Verification items for the finished model (mm, model axes). A direction names the side the tool comes from. Give positions to 0.01 mm unless a question says otherwise; leave off trailing zeros. Order: outer loops, then holes, each group sorted by start corner. A loop starts at its lowest first (then second) coordinate and runs counter-clockwise, first axis right, second up. Notation, with made-up numbers: (29, -31.75) -> (46, -31.75) arc R24 cw to (46, 6.25) -> close; hole circle Ø1 at (81, 78). An arc over 180 degrees is marked (long way). Return JSON: item names as keys, results as strings. Group by question number.
(1) Cross-section at C-C on x = 26.75. Enter the section's corners in (y, z).
(2) Cross-section at D-D on y = 14.5. Enter the section's corners in (x, z).
(3) Cross-section at A-A on x = 14.3. Enter the section's corners in (y, z).
(4) Depth check by flat-ended pin: pin 1 Ø9.5 at (x, z) = (17, 26) entering from -Y; pin 2 Ø3.5 at (x, y) = (11, 15) entering from +Z; pin 3 Ø6 at (x, z) = (10.5, 26) entering from +Y. Enter the tip coordinate at first touch or a pass-through.
(5) Tool access check on faces 1 (the face through (11.1, 10.4, -4.9)), 2 (the face through (14, 13, 26)), 3 (the face through (14, 8, -10)), 4 (the face through (14, 2, 20)). Record the directions out of +Z, -Z, +X, -X, +Y, -Y that give a thin tool (end or side, any length) a straight path to the whole face; none if there is none.
(6) Cross-section at B-B on y = 8. Enter the section's corners in (x, z), then the cut area to 3 significant figures.
(7) Thickness scan on line 1 along Y through (x, z) = (16.75, 25.5); line 2 along Z through (x, y) = (14.5, 12.75); line 3 along Z through (x, y) = (19.25, 14.75). Record the ranges inside material, lowest first.
from build123d import *

# Parameters (mm, degrees)
F0_W     = 28.6
F0_H     = 16
F1_DEPTH = 20
F2_W     = 28.6
F2_H     = 10
F3_DEPTH = 12
F4_R     = 4
F5_DEPTH = 10


with BuildPart() as f1:
    # F0 (on Top) → F1 (new body)
    with BuildSketch(Plane.XY):
        with Locations((14.3, 8)):
            Rectangle(F0_W, F0_H)
    extrude(amount=F1_DEPTH)

    # F2 (on face) → F3 (join)
    with BuildSketch(Plane.XY.offset(20)):
        with Locations((14.3, 8)):
            Rectangle(F2_W, F2_H)
    extrude(amount=F3_DEPTH)

    # F4 (on face) → F5 (join)
    with BuildSketch(Plane(origin=(0, 0, 0), x_dir=(1, 0, 0), z_dir=(0, 0, -1))):
        with Locations((14.3, -8)):
            Circle(F4_R)
    extrude(amount=F5_DEPTH)


solid = f1.part
Verdict:
{
 "1": {"outline": "(0, 0) -> (16, 0) -> (16, 20) -> (13, 20) -> (13, 32) -> (3, 32) -> (3, 20) -> (0, 20) -> close"},
 "2": {"outline": "(0, 0) -> (28.6, 0) -> (28.6, 20) -> (0, 20) -> close"},
 "3": {"outline": "(0, 0) -> (4, 0) -> (4, -10) -> (12, -10) -> (12, 0) -> (16, 0) -> (16, 20) -> (13, 20) -> (13, 32) -> (3, 32) -> (3, 20) -> (0, 20) -> close"},
 "4": {"pin 1": "y = 3", "pin 2": "z = 20", "pin 3": "y = 13"},
 "5": {"face 1": "-Z", "face 2": "+Z, +X, -X, +Y", "face 3": "-Z, +X, -X, +Y, -Y", "face 4": "+Z, +X, -X, -Y"},
 "6": {"outline": "(0, 0) -> (10.3, 0) -> (10.3, -10) -> (18.3, -10) -> (18.3, 0) -> (28.6, 0) -> (28.6, 32) -> (0, 32) -> close", "area": "995 mm²"},
 "7": {"line 1": "3 to 13", "line 2": "0 to 32", "line 3": "0 to 20"}
}
